Check sheet for the modelled part. Datum: model origin and axes. Units: mm. A direction names the side the tool comes from. Coordinates: 2 decimals unless noted, no trailing zeros. Write each loop counter-clockwise with the first axis right and the second up, starting at its lowest first coordinate (ties: lowest second). Pieces come first, ordered by that corner, then holes. Notation, with made-up numbers: (2.25, 36.5) -> (41.25, 36.5) arc R34 cw to (41.25, 72.5) -> close; hole circle Ø4 at (81, 40). An arc over 180 degrees is marked (long way). One line per item, written item: value. Start each with the question number.
1) Sectioned sample at B-B on z = -5. Enter the section's corners in (x, y), plus the area to 3 significant figures.
2) Scan lines: line 1 along Y through (x, z) = (5, 3); line 2 along X through (y, z) = (9.5, 4.5); line 3 along Y through (x, z) = (0, 1.7). Record each from-to range of solid material in increasing order. Write a range as [from, to].
3) Draft check along Y on faces 3 (the cylindrical face through (-5.921, -7.815, 2.535)), 4 (the flat face through (0, 17.5, -11)), 5 (the cylindrical face through (-7.506, 4.521, 2.535)), 6 (the flat face through (-2.5, -15, -10)). Enter one of: +Y half, -Y half, draft (parallel to the pull), parting line (faces both ways), or undercut.
4) Sectioned sample at C-C on x = 0. Give the number of separate pieces and of enclosed holes in the cut face, plus the area to 3 significant figures.
5) Gauge pin test, flat ends, axial feed: P1, Ø1.5, axis at x = 8.66, y = 5, coming from the -Z side; P2, Ø2.5, axis at y = -15.5, z = -6.5, coming from the +X side; P3, Ø3, axis at x = 5, y = -8.66, coming from the -Z side; P4, Ø2.5, axis at y = 14.5, z = -12, coming from the -X side. Record the tip position at first contact, or that the pin passes through.
6) Set-up check for faces 1 (the cylindrical face through (0, -12.5, -11.4)), 2 (the cylindrical face through (4.73, 7.44, 2.54)): record each of +Z, -Z, +X, -X, +Y, -Y from which the full face is reachable in a straight line by a thin tool's end or side.
7) Sectioned sample at A-A on y = 0. Enter the section's corners in (x, z).
8) Sectioned sample at D-D on x = 5.5. Enter the section's corners in (y, z), plus the area to 3 significant figures.
```python
from build123d import *

# Parameters (mm, degrees)
SKETCH1_R           = 12.5
SKETCH1_R_2         = 7.5
BOSS_EXTRUDE1_DEPTH = 5
SKETCH3_R           = 1.25
CUT_EXTRUDE1_DEPTH  = 5
BOSS_EXTRUDE2_START = -30
BOSS_EXTRUDE2_DEPTH = 30
SKETCH6_R           = 1.75
CUT_EXTRUDE2_DEPTH  = 35.003676272
FILLET1_R           = 5
FILLET2_R           = 2.5


with BuildPart() as part:
    # Sketch1 → Boss-Extrude1 (new body)
    with BuildSketch(Plane.XY):
        Circle(SKETCH1_R)
        Circle(SKETCH1_R_2, mode=Mode.SUBTRACT)
    extrude(amount=BOSS_EXTRUDE1_DEPTH)

    # Sketch3 → Cut-Extrude1 (cut)
    with BuildSketch(Plane.XY.offset(5)):
        with Locations((0, 10)):
            Circle(SKETCH3_R)
        with Locations((5, 8.660254038)):
            Circle(SKETCH3_R)
        with Locations((8.660254038, 5)):
            Circle(SKETCH3_R)
        with Locations((10, 0)):
            Circle(SKETCH3_R)
        with Locations((8.660254038, -5)):
            Circle(SKETCH3_R)
        with Locations((5, -8.660254038)):
            Circle(SKETCH3_R)
        with Locations((0, -10)):
            Circle(SKETCH3_R)
        with Locations((-5, -8.660254038)):
            Circle(SKETCH3_R)
        with Locations((-8.660254038, -5)):
            Circle(SKETCH3_R)
        with Locations((-10, 0)):
            Circle(SKETCH3_R)
        with Locations((-8.660254038, 5)):
            Circle(SKETCH3_R)
        with Locations((-5, 8.660254038)):
            Circle(SKETCH3_R)
    extrude(amount=-CUT_EXTRUDE1_DEPTH, mode=Mode.SUBTRACT)

    # Sketch4 → Boss-Extrude2 (add)
    with BuildSketch(Plane.XY.offset(5).offset(BOSS_EXTRUDE2_START)):
        with BuildLine():
            Line((-2.5, 17.5), (-2.5, 12.247448714))
            ThreePointArc((-2.5, 12.247448714), (0, 12.5), (2.5, 12.247448714))
            Line((2.5, 12.247448714), (2.5, 17.5))
            Line((2.5, 17.5), (-2.5, 17.5))
        make_face()
        with BuildLine():
            Line((-2.5, -12.247448714), (-2.5, -17.5))
            Line((-2.5, -17.5), (2.5, -17.5))
            Line((2.5, -17.5), (2.5, -12.247448714))
            ThreePointArc((2.5, -12.247448714), (0, -12.5), (-2.5, -12.247448714))
        make_face()
    extrude(amount=BOSS_EXTRUDE2_DEPTH)

    # Sketch6 → Cut-Extrude2 (cut, through all)
    with BuildSketch(Plane(origin=(2.5, 0, 0), x_dir=(0, 0, -1), z_dir=(1, 0, 0))):
        with Locations((20, 14.873724357)):
            Circle(SKETCH6_R)
        with Locations((20, -14.873724357)):
            Circle(SKETCH6_R)
    extrude(amount=-CUT_EXTRUDE2_DEPTH, mode=Mode.SUBTRACT)

    # Fillet1
    fillet1_edges = [part.edges().sort_by_distance(p)[0] for p in [
        (0, 17.5, 5),
        (0, -17.5, 5),
    ]]
    fillet(fillet1_edges, radius=FILLET1_R)

    # Fillet2
    fillet2_edges = [part.edges().sort_by_distance(p)[0] for p in [
        (0, 12.5, -25),
        (0, 17.5, -25),
        (0, -17.5, -25),
        (0, -12.5, -25),
    ]]
    fillet(fillet2_edges, radius=FILLET2_R - 0.0001)  # a hair under: the kernel refuses the full size


solid = part.part
```
Answers:
1. outline: (-2.5, -17.5) -> (2.5, -17.5) -> (2.5, -12.25) arc R12.5 cw to (-2.5, -12.25) -> close; (-2.5, 12.25) arc R12.5 cw to (2.5, 12.25) -> (2.5, 17.5) -> (-2.5, 17.5) -> close
1. area: 50.8 mm2
2. line 1: y = [-11.46, -9.91], [-7.41, -5.59], [5.59, 7.41], [9.91, 11.46]
2. line 2: x = [-8.12, -5.93], [-4.07, -1.15], [1.15, 4.07], [5.93, 8.12]
2. line 3: y = [-17.2, -11.25], [-8.75, -7.5], [7.5, 8.75], [11.25, 17.2]
3. face 3: undercut
3. face 4: +Y half
3. face 5: undercut
3. face 6: draft
4. separate pieces: 4
4. enclosed holes: 2
4. area: 290 mm2
5. P1: passes through
5. P2: stops at x = 2.5
5. P3: stops at z = 0
5. P4: stops at x = -2.5
6. face 1: -Z
6. face 2: +Z, -Z
7. outline: (-12.5, 0) -> (-11.25, 0) -> (-11.25, 5) -> (-12.5, 5) -> close; (-8.75, 0) -> (-7.5, 0) -> (-7.5, 5) -> (-8.75, 5) -> close; (7.5, 0) -> (8.75, 0) -> (8.75, 5) -> (7.5, 5) -> close; (11.25, 0) -> (12.5, 0) -> (12.5, 5) -> (11.25, 5) -> close
8. outline: (-11.22, 0) -> (-9.81, 0) -> (-9.81, 5) -> (-11.22, 5) -> close; (-7.51, 0) -> (-5.1, 0) -> (-5.1, 5) -> (-7.51, 5) -> close; (5.1, 0) -> (7.51, 0) -> (7.51, 5) -> (5.1, 5) -> close; (9.81, 0) -> (11.22, 0) -> (11.22, 5) -> (9.81, 5) -> close
8. area: 38.3 mm2
